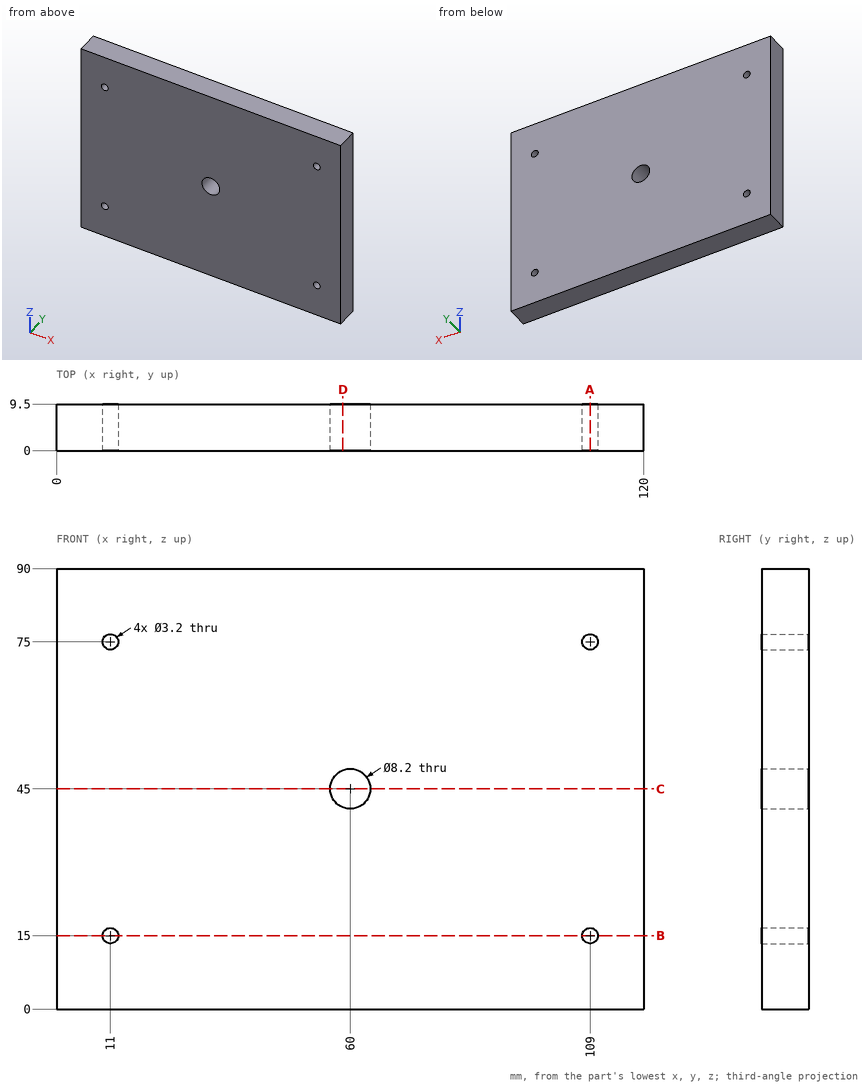
The drawing under review shows one solid part. Ordinate dimensions are in mm from its lowest x, y, z. Round coordinates to 2 decimals unless told otherwise and drop trailing zeros. Loops run counter-clockwise (first coordinate to the right, second up) from the corner with the lowest first, then second, coordinate; pieces in that order, holes last. Notation, with made-up numbers: (20.5, 36) - (69.5, 36) arc R9 ccw to (69.5, 51) - close; hole circle Ø2 at (54.5, -15.5). An arc over 180 degrees is marked (long way). One line per item, written item: value. Start each with the question number.
1) Consider section B-B on z = 15. Give the boundary of the cut face in (x, y).
2) Consider section C-C on z = 45. Give the boundary of the cut face in (x, y).
3) Consider section A-A on x = 109. Give the boundary of the cut face in (y, z), then the cut area to 3 significant figures.
4) Insertion check: pin 1 Ø1.9 at (x, z) = (11, 15) entering from +Y. The pin has a flat end and moves straight along its axis. Give the tip position at first contact, or say it passes through.
5) Consider section D-D on x = 58.5. Give the boundary of the cut face in (y, z).
6) To check wall thickness, follow L1, parallel to Z at x = 109, y = 4.5; L2, parallel to X at y = 4, z = 75; L3, parallel to Z at x = 60, y = 7.75. State the ranges of each line that lie inside material, in increasing order. Write a range as from..to.
Reported:
1. outline: (0, 0) - (9.4, 0) - (9.4, 9.5) - (0, 9.5) - close; (12.6, 0) - (107.4, 0) - (107.4, 9.5) - (12.6, 9.5) - close; (110.6, 0) - (120, 0) - (120, 9.5) - (110.6, 9.5) - close
2. outline: (0, 0) - (55.9, 0) - (55.9, 9.5) - (0, 9.5) - close; (64.1, 0) - (120, 0) - (120, 9.5) - (64.1, 9.5) - close
3. outline: (0, 0) - (9.5, 0) - (9.5, 13.4) - (0, 13.4) - close; (0, 16.6) - (9.5, 16.6) - (9.5, 73.4) - (0, 73.4) - close; (0, 76.6) - (9.5, 76.6) - (9.5, 90) - (0, 90) - close
3. area: 794 mm^2
4. pin 1: passes through
5. outline: (0, 0) - (9.5, 0) - (9.5, 41.18) - (0, 41.18) - close; (0, 48.82) - (9.5, 48.82) - (9.5, 90) - (0, 90) - close
6. L1: z = 0..13.4, 16.6..73.4, 76.6..90
6. L2: x = 0..9.4, 12.6..107.4, 110.6..120
6. L3: z = 0..40.9, 49.1..90
